```python
from build123d import *

# Parameters (mm, degrees)
SKETCH1_W            = 20
SKETCH1_H            = 6
BOSS_EXTRUDE1_DEPTH  = 14.5
SKETCH2_W            = 3
SKETCH2_H            = 20
BOSS_EXTRUDE2_DEPTH  = 12
SKETCH7_R            = 1.5
CUT_EXTRUDE1_DEPTH   = 33.939338184
SKETCH8_R            = 3.4
CUT_EXTRUDE2_DEPTH   = 26.184320519
FILLET1_R            = 3
CONVERT_SOLID3_START = -10
CONVERT_SOLID3_DEPTH = 20


# Read off the part's stored shape, not the designer's step: Convert-Solid3
with BuildPart() as part:
    # Sketch1 → Boss-Extrude1 (new, symmetric)
    with BuildSketch(Plane(origin=(0, 0, 0), x_dir=(0, 0, -1), z_dir=(1, 0, 0))):
        with Locations((0, -3)):
            Rectangle(SKETCH1_W, SKETCH1_H)
    extrude(amount=BOSS_EXTRUDE1_DEPTH, both=True)

    # Sketch2 → Boss-Extrude2 (add)
    with BuildSketch(Plane(origin=(0, 0, 0), x_dir=(1, 0, 0), z_dir=(0, 1, 0))):
        with Locations((13, 0)):
            Rectangle(SKETCH2_W, SKETCH2_H)
        with Locations((-13, 0)):
            Rectangle(SKETCH2_W, SKETCH2_H)
    extrude(amount=BOSS_EXTRUDE2_DEPTH)

    # Sketch7 → Cut-Extrude1 (cut, through all)
    with BuildSketch(Plane.ZY.offset(14.5)):
        with Locations((-5, 7)):
            Circle(SKETCH7_R)
        with Locations((5, 7)):
            Circle(SKETCH7_R)
    extrude(amount=-CUT_EXTRUDE1_DEPTH, mode=Mode.SUBTRACT)

    # Sketch8 → Cut-Extrude2 (cut, through all)
    with BuildSketch(Plane.XZ.offset(6)):
        with Locations(Location((0, 0, 0), (0, 0, 270))):
            Circle(SKETCH8_R)
    extrude(amount=-CUT_EXTRUDE2_DEPTH, mode=Mode.SUBTRACT)

    # Fillet1
    fillet1_edges = [part.edges().sort_by_distance(p)[0] for p in [
        (-13, 12, 10),
        (-13, 12, -10),
        (13, 12, -10),
        (13, 12, 10),
    ]]
    fillet(fillet1_edges, radius=FILLET1_R)

    # Convert-Solid3 outline → Convert-Solid3 (cut)
    with BuildSketch(Plane.XY.offset(CONVERT_SOLID3_START)):
        with BuildLine():
            Line((14.5, -6), (14.5, 0))
            ThreePointArc((14.5, 0), (12.742640687, -4.242640687), (8.5, -6))
            Line((8.5, -6), (14.5, -6))
        make_face()
        with BuildLine():
            Line((-14.5, -6), (-8.5, -6))
            ThreePointArc((-8.5, -6), (-12.742640687, -4.242640687), (-14.5, 0))
            Line((-14.5, 0), (-14.5, -6))
        make_face()
        with BuildLine():
            Line((12.5, 0), (12.5, 12))
            Line((12.5, 12), (11.5, 12))
            Line((11.5, 12), (11.5, 0))
            Line((11.5, 0), (-11.5, 0))
            Line((-11.5, 0), (-11.5, 12))
            Line((-11.5, 12), (-12.5, 12))
            Line((-12.5, 12), (-12.5, 0))
            ThreePointArc((-12.5, 0), (-11.328427125, -2.828427125), (-8.5, -4))
            Line((-8.5, -4), (8.5, -4))
            ThreePointArc((8.5, -4), (11.328427125, -2.828427125), (12.5, 0))
        make_face()
    extrude(amount=CONVERT_SOLID3_DEPTH, mode=Mode.SUBTRACT)


solid = part.part
```
Geometry check sheet. Reference: the model listing, model coordinates, mm. A direction names the side the tool comes from. Round coordinates to 2 decimals unless told otherwise and drop trailing zeros. Loops run counter-clockwise (first coordinate to the right, second up) from the corner with the lowest first, then second, coordinate; pieces in that order, holes last. Notation, with made-up numbers: (34, 32) - (87, 32) arc R9 ccw to (87, 37) - close; hole circle Ø6 at (-25.75, 27.25). An arc over 180 degrees is marked (long way). Write item = value, one per line. Start each with the question number.
1. Section check C-C on y = 7. Enter the section's corners in (x, z).
2. Section check A-A on z = 5. Enter the section's corners in (x, y).
3. Depth check by flat-ended pin: pin 1 (2.5 mm diameter, centred on y = 7, z = -5, fed in from -X); pin 2 (10 mm diameter, centred on x = -6.5, z = -7.5, fed in from +Y); pin 3 (1 mm diameter, centred on x = -7, z = 0, fed in from +Y); pin 4 (2 mm diameter, centred on y = -4, z = 6, fed in from -X). Enter the tip coordinate at first touch or a pass-through.
4. Mould release check, pull along X, two halves, no side actions. Record for faces 3 (the face through (13.49, 5.67, 5.69)), 4 (the face through (11.297, -2.859, -0.14)), 5 (the face through (-14.5, 6, 0)), 6 (the face through (12.789, -4.196, -0.14)): released by +X, released by -X, zero draft, split by the parting line, or undercut.
5. Section check B-B on x = 0. Enter the section's corners in (y, z), then the cut area to 3 significant figures.
6. Section check D-D on z = 0. Enter the section's corners in (x, y).
7. Set-up check for faces 1 (the face through (0, -5, -10)), 2 (the face through (4, -4, 0)): record each of +Z, -Z, +X, -X, +Y, -Y from which the full face is reachable in a straight line by a thin tool's end or side.
8. Thickness scan on line 1 (X direction, y = 9.5, z = -7.25); line 2 (Y direction, x = -13.25, z = 5); line 3 (X direction, y = -1, z = 3). Record the ranges inside material, lowest first.
Working result:
q1.outline = (-14.5, -10) - (-12.5, -10) - (-12.5, -6.5) - (-14.5, -6.5) - close; (-14.5, -3.5) - (-12.5, -3.5) - (-12.5, 3.5) - (-14.5, 3.5) - close; (-14.5, 6.5) - (-12.5, 6.5) - (-12.5, 10) - (-14.5, 10) - close; (12.5, -10) - (14.5, -10) - (14.5, -6.5) - (12.5, -6.5) - close; (12.5, -3.5) - (14.5, -3.5) - (14.5, 3.5) - (12.5, 3.5) - close; (12.5, 6.5) - (14.5, 6.5) - (14.5, 10) - (12.5, 10) - close
q2.outline = (-14.5, 0) arc R6 ccw to (-8.5, -6) - (8.5, -6) arc R6 ccw to (14.5, 0) - (14.5, 5.5) - (12.5, 5.5) - (12.5, 0) arc R4 cw to (8.5, -4) - (-8.5, -4) arc R4 cw to (-12.5, 0) - (-12.5, 5.5) - (-14.5, 5.5) - close; (-14.5, 8.5) - (-12.5, 8.5) - (-12.5, 12) - (-14.5, 12) - close; (12.5, 8.5) - (14.5, 8.5) - (14.5, 12) - (12.5, 12) - close
q3.pin_1 = through
q3.pin_2 = -2.65
q3.pin_3 = -4
q3.pin_4 = -13.7
q4.face_3 = zero draft
q4.face_4 = undercut
q4.face_5 = released by -X
q4.face_6 = released by +X
q5.outline = (-6, -10) - (-4, -10) - (-4, -3.4) - (-6, -3.4) - close; (-6, 3.4) - (-4, 3.4) - (-4, 10) - (-6, 10) - close
q5.area = 26.4 mm^2
q6.outline = (-14.5, 0) arc R6 ccw to (-8.5, -6) - (-3.4, -6) - (-3.4, -4) - (-8.5, -4) arc R4 cw to (-12.5, 0) - (-12.5, 12) - (-14.5, 12) - close; (3.4, -6) - (8.5, -6) arc R6 ccw to (14.5, 0) - (14.5, 12) - (12.5, 12) - (12.5, 0) arc R4 cw to (8.5, -4) - (3.4, -4) - close
q7.face_1 = -Z, +X, -X, +Y, -Y
q7.face_2 = +Z, -Z, +Y
q8.line_1 = -14.5 to -12.5, 12.5 to 14.5
q8.line_2 = -3.67 to 5.5, 8.5 to 12
q8.line_3 = -14.42 to -12.37, 12.37 to 14.42
